```python
from build123d import *

# Parameters (mm, degrees)
SKETCH_W     = 54
SKETCH_H     = 29
SKETCH_W_2   = 50
SKETCH_H_2   = 25
PAD_DEPTH    = 30
POCKET_DEPTH = 54.001
PAD001_DEPTH = 52


with BuildPart() as part:
    # Sketch → Pad (new body)
    with BuildSketch(Plane.XY):
        with Locations((27, 14.5)):
            Rectangle(SKETCH_W, SKETCH_H)
        with Locations((27, 14.5)):
            Rectangle(SKETCH_W_2, SKETCH_H_2, mode=Mode.SUBTRACT)
    extrude(amount=PAD_DEPTH)

    # Sketch001 (on Face2 of Pad) → Pocket (cut, through all)
    with BuildSketch(Plane.YZ.offset(54)):
        with BuildLine():
            ThreePointArc((24.5, 0), (14.5, 10), (4.5, 0))
            Line((4.5, 0), (24.5, 0))
        make_face()
    extrude(amount=-POCKET_DEPTH, mode=Mode.SUBTRACT)

    # Sketch002 (on Face3 of Pocket) → Pad001 (join)
    with BuildSketch(Plane.YZ.offset(54)):
        with BuildLine():
            ThreePointArc((24.5, 0), (14.5, 10), (4.5, 0))
            Line((0, 0), (4.5, 0))
            Line((0, 0), (0, 2))
            Line((0, 2), (2.66784, 2))
            ThreePointArc((26.33216, 2), (14.5, 12), (2.66784, 2))
            Line((29, 2), (26.33216, 2))
            Line((29, 0), (29, 2))
            Line((24.5, 0), (29, 0))
        make_face()
    extrude(amount=-PAD001_DEPTH)


solid = part.part
```
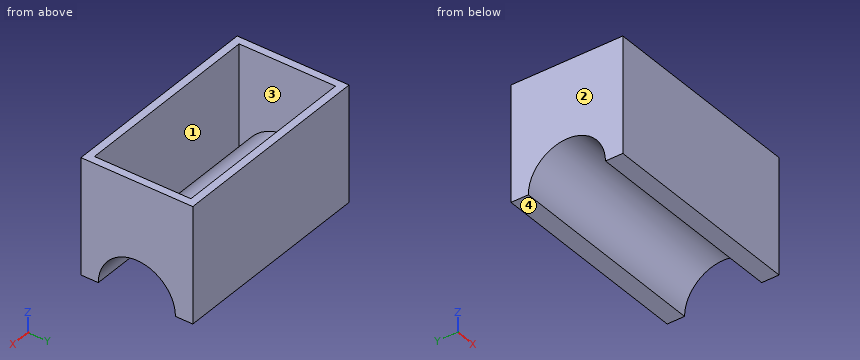
Can you work these out from the model? Positions are in its coordinate system, mm. Face numbers are marked on the shaded views. Give positions to 0.01 mm unless a question says otherwise; leave off trailing zeros. Order: outer loops, then holes, each group sorted by start corner. A loop starts at its lowest first (then second) coordinate and runs counter-clockwise, first axis right, second up. Notation, with made-up numbers: M 73.25,73 L 85.25,73 A33 cw 85.25,103 Z; hole C -12.75,-24.75 d8. An arc over 180 degrees is marked long. Write item = value, one per line. Start each with the question number.
Q1. Suppose I cut it at A-A (x = 15.5). Write out the boundary of the cut face in (y, z).
Q2. Suppose I cut it at B-B (z = 9.25). Write out the boundary of the cut face in (x, y).
Q3. I need wall thicknesses on probe 1 along X at (y, z) = (18, 27); probe 2 along Y at (x, z) = (46.5, 27.75); probe 3 along Y at (x, z) = (33, 3.75). Which ranges of each line are inside material? Lowest first, please. Write a range as [from, to].
Q4. We'd pull the mould along X, two halves only. Please class the marked faces 1, 2, 3 and 4: pulls with the +X half, pulls with the -X half, needs draft (parallel to the pull), parting line crosses it, or undercut.
Q5. Will this pin go through, and if not, where does the flat tip stop? pin 1 Ø3 at (x, y) = (46, 13) entering from -Z.
Q6. Suppose I cut it at D-D (z = 16). Write out the boundary of the cut face in (x, y), plus the area to 3 significant figures.
Q7. Suppose I cut it at C-C (y = 14.5). Write out the boundary of the cut face in (x, z).
Check result:
q1.outline = M 0,0 L 4.5,0 A10 cw 24.5,0 L 29,0 L 29,30 L 27,30 L 27,2 L 26.33,2 A12 ccw 2.67,2 L 2,2 L 2,30 L 0,30 Z
q2.outline = M 0,0 L 54,0 L 54,10.7 L 0,10.7 Z; M 0,18.3 L 54,18.3 L 54,29 L 0,29 Z; hole M 2,2 L 52,2 L 52,6.86 L 2,6.86 Z; hole M 2,22.14 L 52,22.14 L 52,27 L 2,27 Z
q3.probe_1 = [0, 2], [52, 54]
q3.probe_2 = [0, 2], [27, 29]
q3.probe_3 = [0, 2], [3.1, 5.23], [23.77, 25.9], [27, 29]
q4.face_1 = undercut
q4.face_2 = pulls with the -X half
q4.face_3 = undercut
q4.face_4 = needs draft
q5.pin_1 = 9.54
q6.outline = M 0,0 L 54,0 L 54,29 L 0,29 Z; hole M 2,2 L 52,2 L 52,27 L 2,27 Z
q6.area = 316 mm2
q7.outline = M 0,10 L 54,10 L 54,30 L 52,30 L 52,12 L 2,12 L 2,30 L 0,30 Z
